Autodesk Inventor part; units mm, degrees
ref_plane "YZ Plane" through (0, 0, 0) normal (1, 0, 0) x (0, 1, 0)
ref_plane "XZ Plane" through (0, 0, 0) normal (0, 1, 0) x (-1, 0, 0)
ref_plane "XY Plane" through (0, 0, 0) normal (0, 0, 1) x (1, 0, 0)
sketch "Sketch1" plane through (0, 0, 0) normal (0, 0, 1) x (1, 0, 0)
  line L0 (0, 247.65) -> (0, -247.65) construction
  line L1 (-44.45, 247.65) -> (-44.45, -247.65)
  line L2 (44.45, -247.65) -> (44.45, 247.65)
  arc A0 (44.45, 247.65) -> (-44.45, 247.65) centre (0, 247.65) ccw
  arc A1 (-44.45, -247.65) -> (44.45, -247.65) centre (0, -247.65) ccw
  line L3 (-42.8625, -247.65) -> (-42.8625, 247.65)
  arc A2 (42.8625, 247.65) -> (-42.8625, 247.65) centre (0, 247.65) ccw
  line L4 (42.8625, 247.65) -> (42.8625, -247.65)
  arc A3 (-42.8625, -247.65) -> (42.8625, -247.65) centre (0, -247.65) ccw
  point P0 (0, 0)
  dimension "d0" = 495.3
  dimension "d1" = 44.45
  dimension "d2" = 1.5875
extrude "Extrusion1" add sketch "Sketch1" along normal mid plane 50.8
properties part number "1_16 Thick x 2 Wide Urethane Flat Belting (10 Long)(217-6002)" material "Rubber"
The listing builds one solid part. Answer for the finished solid, in the listing's coordinates (mm). A direction names the side the tool comes from. Round coordinates to 2 decimals unless told otherwise and drop trailing zeros. Write each loop counter-clockwise with the first axis right and the second up, starting at its lowest first coordinate (ties: lowest second). Pieces come first, ordered by that corner, then holes. Notation, with made-up numbers: (-30, 39) - (-24, 39) arc R14 cw to (-24, 66) - close; hole circle Ø3 at (24.5, 20.25). An arc over 180 degrees is marked (long way). Use a Markdown table: item, result. Add a question column.
1. The part is cut by section A-A (y = -187.5). Write down the section's boundary in (x, z), and give its area (3 significant figures).
2. For a pull along X with two mould halves and no side action, classify faces 3 (the face through (0.98, -292.09, -0.36)), 4 (the face through (-44.45, 3, 0)), 5 (the face through (-0.943, 290.502, -0.356)) as +X half, -X half, draft (parallel to the pull), parting line (faces both ways), or undercut.
3. The part is cut by section B-B (x = 0). Write down the section's boundary in (y, z).
4. Consider line 1 (X direction, y = 118, z = -10.5); line 2 (Y direction, x = 0, z = -7); line 3 (Y direction, x = -15, z = 10.5). Determine where each line is inside the solid, lowest interval first.
5. Flat-ended cylindrical pins translate along their axes: P1, Ø12, axis at x = 31, z = 15, coming from the +Y side; P2, Ø3, axis at x = 25.5, z = 14.5, coming from the +Y side; P3, Ø10, axis at x = 28.5, z = -4, coming from the -Y side. Find the tip coordinate at first contact, or state that the pin passes through.
6. A tool of negligible diameter and unlimited length cuts with its end or side. For faces 1 (the face through (42.862, 3, 0)), 2 (the face through (44.45, -3, 0)), from which of +Z, -Z, +X, -X, +Y, -Y can it reach the whole face along a straight path? Write none if from no direction.
Reported:
| question | item | result |
|---|---|---|
| 1 | outline | (-44.45, -25.4) - (-42.86, -25.4) - (-42.86, 25.4) - (-44.45, 25.4) - close; (42.86, -25.4) - (44.45, -25.4) - (44.45, 25.4) - (42.86, 25.4) - close |
| 1 | area | 161 mm^2 |
| 2 | face 3 | parting line |
| 2 | face 4 | -X half |
| 2 | face 5 | undercut |
| 3 | outline | (-292.1, -25.4) - (-290.51, -25.4) - (-290.51, 25.4) - (-292.1, 25.4) - close; (290.51, -25.4) - (292.1, -25.4) - (292.1, 25.4) - (290.51, 25.4) - close |
| 4 | line 1 | -44.45 to -42.86, 42.86 to 44.45 |
| 4 | line 2 | -292.1 to -290.51, 290.51 to 292.1 |
| 4 | line 3 | -289.49 to -287.8, 287.8 to 289.49 |
| 5 | P1 | y = 284.4 |
| 5 | P2 | y = 285.06 |
| 5 | P3 | y = -285.38 |
| 6 | face 1 | +Z, -Z |
| 6 | face 2 | +Z, -Z, +X, +Y, -Y |
